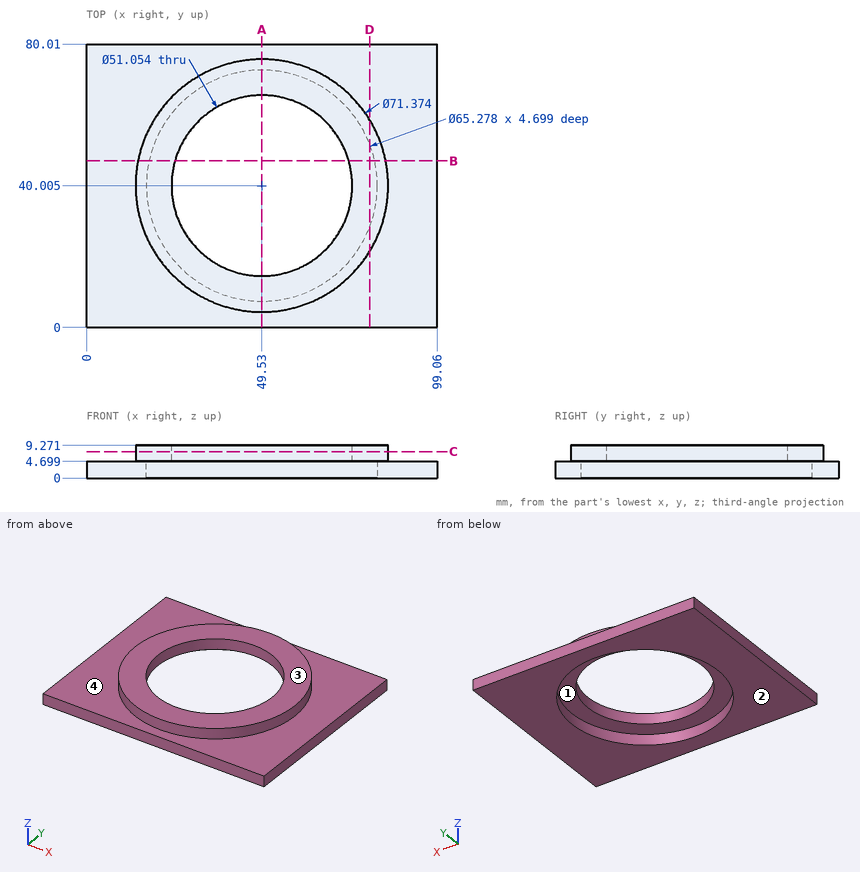
Study the drawing (mm; zero at the part's minimum x, y, z) and answer. A direction names the side the tool comes from. Give positions to 0.01 mm unless a question says otherwise; leave off trailing zeros. Write each loop counter-clockwise with the first axis right and the second up, starting at its lowest first coordinate (ties: lowest second). Pieces come first, ordered by that corner, then holes.
(1) The mould has two halves that part along Y. Classify the marked faces 1 and 2: pulls with the +Y half, pulls with the -Y half, needs draft (parallel to the pull), parting line crosses it, or undercut.
Final values:
face 1: undercut
face 2: needs draft
(2) The part is cut by section A-A on x = 49.53. Write down the section's boundary in (y, z).
Final values:
outline: (0, 0) - (7.37, 0) - (7.37, 4.7) - (14.48, 4.7) - (14.48, 9.27) - (4.32, 9.27) - (4.32, 4.7) - (0, 4.7) - close; (65.53, 4.7) - (72.64, 4.7) - (72.64, 0) - (80.01, 0) - (80.01, 4.7) - (75.69, 4.7) - (75.69, 9.27) - (65.53, 9.27) - close
(3) Flat-ended cylindrical pins translate along their axes: pin 1 Ø3 at (y, z) = (43.5, 8) entering from +X; pin 2 Ø4 at (x, y) = (50, 12) entering from -Z; pin 3 Ø2 at (x, y) = (68.5, 71.5) entering from +Z. Find the tip coordinate at first contact, or state that the pin passes through.
Final values:
pin 1: stops at x = 85.16
pin 2: stops at z = 4.7
pin 3: stops at z = 4.7
(4) The part is cut by section D-D on x = 80. Write down the section's boundary in (y, z).
Final values:
outline: (0, 0) - (28.31, 0) - (28.31, 4.7) - (51.7, 4.7) - (51.7, 0) - (80.01, 0) - (80.01, 4.7) - (58.58, 4.7) - (58.58, 9.27) - (21.43, 9.27) - (21.43, 4.7) - (0, 4.7) - close
(5) Which of the six approach directions +Z, -Z, +X, -X, +Y, -Y give full straight-line access (tool end or side, diameter ignored) to the marked faces 3 and 4?
Final values:
face 3: +Z, +X, -X, +Y, -Y
face 4: +Z
(6) The part is cut by section C-C on z = 7.5. Write down the section's boundary in (x, y) (3 decimals), plus the area to 3 significant figures.
Final values:
outline: circle Ø71.374 at (49.53, 40.005); hole circle Ø51.054 at (49.53, 40.005)
area: 1,950 mm2
(7) Straight lines are drawn through the part: line 1 (Y direction, x = 49.53, z = 6.9); line 2 (Y direction, x = 49.53, z = 1.05); line 3 (Z direction, x = 80.5, y = 72.5). For each, find the intervals that lie inside material, in ascending order.
Final values:
line 1: y = 4.32 to 14.48, 65.53 to 75.69
line 2: y = 0 to 7.37, 72.64 to 80.01
line 3: z = 0 to 4.7
(8) The part is cut by section B-B on y = 47. Write down the section's boundary in (x, z).
Final values:
outline: (0, 0) - (17.65, 0) - (17.65, 4.7) - (24.98, 4.7) - (24.98, 9.27) - (14.54, 9.27) - (14.54, 4.7) - (0, 4.7) - close; (74.08, 4.7) - (81.41, 4.7) - (81.41, 0) - (99.06, 0) - (99.06, 4.7) - (84.52, 4.7) - (84.52, 9.27) - (74.08, 9.27) - close
